from build123d import *

# Parameters (mm, degrees)
SKETCH1_W                 = 25.4
SKETCH1_H                 = 38.1
BOSS_EXTRUDE1_DEPTH       = 9.525
F_1_4_CLEARANCE_HOLE1_D   = 6.7564
F_8_32_TAPPED_HOLE1_D     = 3.4544
F_8_32_TAPPED_HOLE1_DEPTH = 10.668
F_8_32_TAPPED_HOLE1_TIP   = 1.037806461


with BuildPart() as part:
    # Sketch1 → Boss-Extrude1 (new, symmetric)
    with BuildSketch(Plane(origin=(0, 0, 0), x_dir=(1, 0, 0), z_dir=(0, 1, 0))):
        Rectangle(SKETCH1_W, SKETCH1_H)
    extrude(amount=BOSS_EXTRUDE1_DEPTH, both=True)

    # 1/4 Clearance Hole1 (through all)
    with Locations(Plane.XY.offset(19.05)):
        with Locations((0, 0)):
            Hole(F_1_4_CLEARANCE_HOLE1_D / 2)

    # #8-32 Tapped Hole1
    with Locations(Plane(origin=(0, -9.525, 0), x_dir=(-1, 0, 0), z_dir=(0, -1, 0))):
        with Locations((8.89, -12.7), (-8.89, 12.7)):
            Hole(F_8_32_TAPPED_HOLE1_D / 2, depth=F_8_32_TAPPED_HOLE1_DEPTH)
            with Locations((0, 0, -(F_8_32_TAPPED_HOLE1_DEPTH + F_8_32_TAPPED_HOLE1_TIP / 2))):  # 118° drill point
                Cone(0, F_8_32_TAPPED_HOLE1_D / 2, F_8_32_TAPPED_HOLE1_TIP, mode=Mode.SUBTRACT)


solid = part.part
Model file for the job. Use its own axes, mm. A direction names the side the tool comes from. Give positions to 0.01 mm unless a question says otherwise; leave off trailing zeros. Loops run counter-clockwise (first coordinate to the right, second up) from the corner with the lowest first, then second, coordinate; pieces in that order, holes last.
Item 1: Slice it at C-C (x = 0). Write the cut outline in (y, z) (3 decimals), plus the area to 3 significant figures.
Check values:
outline: (-9.525, -19.05) - (-3.378, -19.05) - (-3.378, 19.05) - (-9.525, 19.05) - close; (3.378, -19.05) - (9.525, -19.05) - (9.525, 19.05) - (3.378, 19.05) - close
area: 468 mm2
Item 2: Which spindle directions (+Z, -Z, +X, -X, +Y, -Y) get a long thin tool onto all of the face, cutting with end or side? Do faces 5 (the face through (7.52, -4.12, -11.65)), 6 (the face through (0, 9.525, 0)). Say none if no direction does.
Check values:
face 5: -Y
face 6: +Z, -Z, +X, -X, +Y
Item 3: Slice it at D-D (y = -4.75). Write the cut outline in (x, z), plus the area to 3 significant figures.
Check values:
outline: (-12.7, -19.05) - (12.7, -19.05) - (12.7, 19.05) - (-12.7, 19.05) - close; hole circle Ø3.45 at (-8.89, 12.7); hole circle Ø3.45 at (8.89, -12.7)
area: 949 mm2
Item 4: Mould opens along Z. For faces 1 (the face through (-3, 2, 19.05)), 2 (the face through (-12.7, 0, 0)), 3 (the face through (-3, 2, -19.05)), 4 (the face through (-10.616, -4.116, 12.624)) say: +Z half, -Z half, draft (parallel to the pull), parting line (faces both ways), or undercut.
Check values:
face 1: +Z half
face 2: draft
face 3: -Z half
face 4: undercut
Item 5: Slice it at A-A (y = 0). Write the cut outline in (x, z), plus the area to 3 significant figures.
Check values:
outline: (-12.7, -19.05) - (-3.38, -19.05) - (-3.38, 19.05) - (-12.7, 19.05) - close; (3.38, -19.05) - (12.7, -19.05) - (12.7, 19.05) - (3.38, 19.05) - close; hole circle Ø3.45 at (-8.89, 12.7); hole circle Ø3.45 at (8.89, -12.7)
area: 692 mm2
Item 6: Drill centre lines: line 1 along Z through (x, y) = (-8.89, -5); line 2 along X through (y, z) = (-1.75, 12.7); line 3 along X through (y, z) = (0.5, -13). Where is each one in solid material? Low to high.
Check values:
line 1: z = -19.05 to 10.97, 14.43 to 19.05
line 2: x = -12.7 to -10.62, -7.16 to -2.89, 2.89 to 12.7
line 3: x = -12.7 to -3.34, 3.34 to 7.19, 10.59 to 12.7
Item 7: Slice it at B-B (z = -6.5). Write the cut outline in (x, y) (3 decimals).
Check values:
outline: (-12.7, -9.525) - (12.7, -9.525) - (12.7, 9.525) - (-12.7, 9.525) - close; hole circle Ø6.756 at (0, 0)
